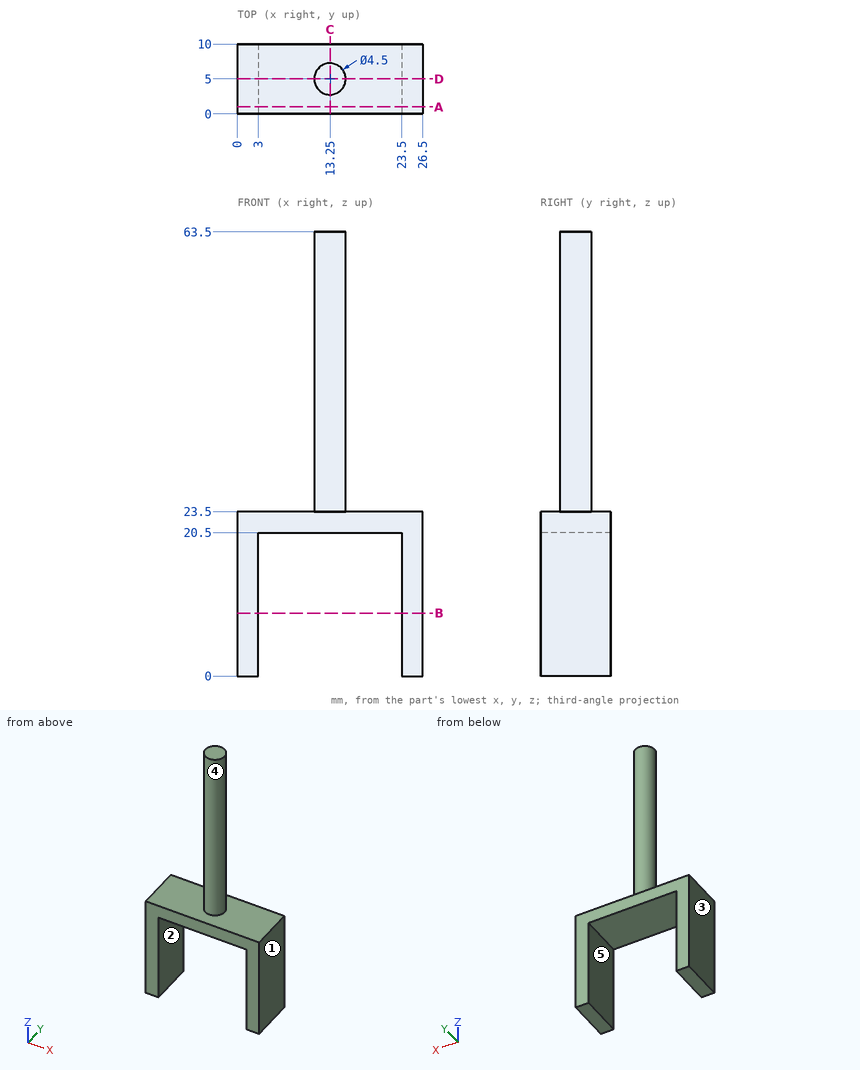
Design review of the part shown in the three views and the two pictorial views. Dimensions are in mm from the part's minimum x, y and z. A direction names the side the tool comes from. Round coordinates to 2 decimals unless told otherwise and drop trailing zeros. Order: outer loops, then holes, each group sorted by start corner. A loop starts at its lowest first (then second) coordinate and runs counter-clockwise, first axis right, second up. Notation, with made-up numbers: (-29, -39.75) - (1, -39.75) arc R11 ccw to (1, -34.75) - close; hole circle Ø11 at (46.25, -17.5). An arc over 180 degrees is marked (long way). Answer in a Markdown table with one row per item.
(1) Take a section at B-B on z = 9. Write out the cut boundary in (x, y), plus the area to 3 significant figures.
Result set:
| item | result |
|---|---|
| outline | (0, 0) - (3, 0) - (3, 10) - (0, 10) - close; (23.5, 0) - (26.5, 0) - (26.5, 10) - (23.5, 10) - close |
| area | 60.0 mm2 |
(2) Take a section at A-A on y = 1. Write out the cut boundary in (x, z).
Result set:
| item | result |
|---|---|
| outline | (0, 0) - (3, 0) - (3, 20.5) - (23.5, 20.5) - (23.5, 0) - (26.5, 0) - (26.5, 23.5) - (0, 23.5) - close |
(3) Clearance check with flat-ended pins moving along their axes: P1, Ø1, axis at x = 3, z = 10.5, coming from the -Y side; P2, Ø6, axis at x = 15.5, z = 32.5, coming from the +Y side. State where each tip first meets the part, or that it passes through.
Result set:
| item | result |
|---|---|
| P1 | stops at y = 0 |
| P2 | stops at y = 7.25 |
(4) Take a section at D-D on y = 5. Write out the cut boundary in (x, z), plus the area to 4 significant figures.
Result set:
| item | result |
|---|---|
| outline | (0, 0) - (3, 0) - (3, 20.5) - (23.5, 20.5) - (23.5, 0) - (26.5, 0) - (26.5, 23.5) - (15.5, 23.5) - (15.5, 63.5) - (11, 63.5) - (11, 23.5) - (0, 23.5) - close |
| area | 382.5 mm2 |
(5) Mouldability with a two-part tool opening along X and no side actions: class the marked faces 3, 4 and 5 as released by +X, released by -X, zero draft, split by the parting line, or undercut.
Result set:
| item | result |
|---|---|
| face 3 | released by -X |
| face 4 | split by the parting line |
| face 5 | undercut |
(6) Take a section at C-C on x = 13.25. Write out the cut boundary in (y, z).
Result set:
| item | result |
|---|---|
| outline | (0, 20.5) - (10, 20.5) - (10, 23.5) - (7.25, 23.5) - (7.25, 63.5) - (2.75, 63.5) - (2.75, 23.5) - (0, 23.5) - close |
(7) For line 1 (X direction, y = 1.25, z = 14); line 2 (Z direction, x = 8, y = 6); line 3 (Z direction, x = 1.5, y = 1.25), list the stretches that pass through material, from the lowest coordinate up. Write a range as from..to.
Result set:
| item | result |
|---|---|
| line 1 | x = 0..3, 23.5..26.5 |
| line 2 | z = 20.5..23.5 |
| line 3 | z = 0..23.5 |
(8) Machinability: for the marked faces 1 and 2, which of the approach directions +Z, -Z, +X, -X, +Y, -Y give a long, thin tool a straight path to every point of the face, cutting with its end or side? Answer none if there is none.
Result set:
| item | result |
|---|---|
| face 1 | +Z, -Z, +X, +Y, -Y |
| face 2 | -Z, +Y, -Y |
